Check sheet for the modelled part. Datum: model origin and axes. Units: mm. A direction names the side the tool comes from. Round coordinates to 2 decimals unless told otherwise and drop trailing zeros. Order: outer loops, then holes, each group sorted by start corner. A loop starts at its lowest first (then second) coordinate and runs counter-clockwise, first axis right, second up.
Q1. Cross-section at C-C on y = 0. Record the cut outline in (x, z), then the cut area to 3 significant figures.
Q2. Depth check by flat-ended pin: P1, Ø1.5, axis at x = -15, z = 4, coming from the -Y side; P2, Ø2, axis at x = -6.5, z = 3.5, coming from the +Y side; P3, Ø1.5, axis at y = 25, z = 1, coming from the +X side. Enter the tip coordinate at first touch or a pass-through.
Q3. Cross-section at A-A on z = 1.15. Record the cut outline in (x, y).
Q4. Mould release check, pull along Y, two halves, no side actions. Record for faces 5 (the flat face through (-4.247, 4.327, 2.465)), 6 (the cylindrical face through (-7.13, -32.12, 2.46)), 7 (the flat face through (1.62, 5.84, 2.46)), 8 (the flat face through (0, -7, 5)): +Y half, -Y half, draft (parallel to the pull), parting line (faces both ways), or undercut.
Q5. Cross-section at B-B on x = 0. Record the cut outline in (y, z), then the cut area to 3 significant figures.
Q6. Cross-section at D-D on y = -19. Record the cut outline in (x, z).
Q7. Scan lines: probe 1 along Y at (x, z) = (1.5, 2.55); probe 2 along Z at (x, y) = (27.5, -13); probe 3 along Y at (x, z) = (-4, 0.5). Record each from-to range of solid material in increasing order.
Q8. Set-up check for faces 1 (the flat face through (26, -16, 3.5)), 2 (the flat face through (5.87, 1.51, 2.46)), 3 (the flat face through (-23.605, 19.181, 4.24)), 4 (the flat face through (23.605, -19.181, 4.24)): record each of +Z, -Z, +X, -X, +Y, -Y from which the full face is reachable in a straight line by a thin tool's end or side.
from build123d import *

# Parameters (mm, degrees)
SKETCH_1_R               = 32.9
EXTRUDE_1_DEPTH          = 5
CUT_EXTRUDE_START        = -1.5
CUT_EXTRUDE_1_DEPTH      = 1.5
PATTERN_CIRCULAR_1_COUNT = 2


with BuildPart() as part:
    # 草图1 → 凸台-拉伸1 (new body)
    with BuildSketch(Plane.XY):
        Circle(SKETCH_1_R)
        Polygon((6.759189323, -1.820263634), (4.95598921, 4.943497845), (-1.803200113, 6.76376148), (-6.759189323, 1.820263634), (-4.95598921, -4.943497845), (1.803200113, -6.76376148), align=None, mode=Mode.SUBTRACT)
    extrude(amount=EXTRUDE_1_DEPTH)

    # 草图2 → 切除-拉伸1 (cut)
    with BuildSketch(Plane.XY.offset(5).offset(CUT_EXTRUDE_START)):
        with BuildLine():
            Line((-30.032915542, 13.432571759), (-25.559928121, 11.431975965))
            ThreePointArc((-25.559928121, 11.431975965), (-23.8490871, 14.670413917), (-21.730181587, 17.657837019))
            Line((-21.730181587, 17.657837019), (-25.532963365, 20.747958497))
            ThreePointArc((-25.532963365, 20.747958497), (-28.022677343, 17.237736352), (-30.032915542, 13.432571759))
        make_face()
    cut_extrude_1 = extrude(amount=CUT_EXTRUDE_1_DEPTH, mode=Mode.SUBTRACT)

    # 阵列(圆周)1: 切除-拉伸1 ×2 about axis
    pattern_circular_1_axis = Axis((0, 0, 0), (0, 0, 1))
    for i in range(1, PATTERN_CIRCULAR_1_COUNT):
        add(cut_extrude_1.rotate(pattern_circular_1_axis, i * 360 / PATTERN_CIRCULAR_1_COUNT), mode=Mode.SUBTRACT)


solid = part.part
Results found:
1. outline: (-32.9, 0) - (-6.27, 0) - (-6.27, 5) - (-32.9, 5) - close; (6.27, 0) - (32.9, 0) - (32.9, 5) - (6.27, 5) - close
1. area: 266 mm2
2. P1: stops at y = -29.65
2. P2: stops at y = 32.44
2. P3: stops at x = 22.23
3. outline: circle Ø65.8 at (0, 0); hole (-6.76, 1.82) - (-4.96, -4.94) - (1.8, -6.76) - (6.76, -1.82) - (4.96, 4.94) - (-1.8, 6.76) - close
4. face 5: undercut
4. face 6: parting line
4. face 7: undercut
4. face 8: draft
5. outline: (-32.9, 0) - (-6.28, 0) - (-6.28, 5) - (-32.9, 5) - close; (6.28, 0) - (32.9, 0) - (32.9, 5) - (6.28, 5) - close
5. area: 266 mm2
6. outline: (-26.86, 0) - (26.86, 0) - (26.86, 3.5) - (23.38, 3.5) - (23.38, 5) - (-26.86, 5) - close
7. probe 1: y = -32.87 to -6.68, 5.87 to 32.87
7. probe 2: z = 0 to 3.5
7. probe 3: y = -32.66 to -5.2, 4.57 to 32.66
8. face 1: +Z
8. face 2: +Z, -Z
8. face 3: +Z, -X
8. face 4: +Z, +X
